from build123d import *

# Parameters (mm, degrees)
F0_R      = 8.25
F1_DEPTH  = 7
F2_R      = 3
F3_DEPTH  = 1
F4_R      = 5.75
F5_DEPTH  = 1.25
F6_R      = 3.35
F7_DEPTH  = 5.5
F9_DEPTH  = 5.5
F10_R     = 2
F11_DEPTH = 25
F13_DEPTH = 2.5


with BuildPart() as f1:
    # F0 (on Top) → F1 (new body)
    with BuildSketch(Plane.XY):
        Circle(F0_R)
    extrude(amount=F1_DEPTH)

    # F2 (on face) → F3 (join)
    with BuildSketch(Plane(origin=(0, 0, 0), x_dir=(1, 0, 0), z_dir=(0, 0, -1))):
        Circle(F2_R)
    extrude(amount=F3_DEPTH)

    # F4 (on face) → F5 (join)
    with BuildSketch(Plane.XY.offset(7)):
        Circle(F4_R)
    extrude(amount=F5_DEPTH)

    # F6 (on face) → F7 (join)
    with BuildSketch(Plane.XY.offset(8.25)):
        Circle(F6_R)
    extrude(amount=F7_DEPTH)

    # F8 (on face) → F9 (cut, through all)
    with BuildSketch(Plane.XY.offset(13.75)):
        with BuildLine():
            ThreePointArc((-2.9, 1.677051), (-3.35, 0), (-2.9, -1.677051))
            Line((-2.9, -1.677051), (-2.9, 1.677051))
        make_face()
        with BuildLine():
            Line((2.9, 1.677051), (2.9, -1.677051))
            ThreePointArc((2.9, -1.677051), (3.235545, -0.868188), (3.35, 0))
            ThreePointArc((3.35, 0), (3.235545, 0.868188), (2.9, 1.677051))
        make_face()
    extrude(amount=-F9_DEPTH, mode=Mode.SUBTRACT)

    # F10 (on face) → F11 (join)
    with BuildSketch(Plane.XY.offset(13.75)):
        Circle(F10_R)
    extrude(amount=F11_DEPTH)

    # F12 (on face) → F13 (join)
    with BuildSketch(Plane.XY.offset(7)):
        Polygon((-8.5, -11.45), (8.5, -11.45), (8.5, -6.003058), (6.946942, -4.45), (-6.946942, -4.45), (-8.5, -6.003058), align=None)
    extrude(amount=-F13_DEPTH)


solid = f1.part
Read the model definition and answer for the solid it produces. Units are mm, in the model's axes. A direction names the side the tool comes from. Coordinates: 2 decimals unless noted, no trailing zeros. Loops run counter-clockwise (first coordinate to the right, second up) from the corner with the lowest first, then second, coordinate; pieces in that order, holes last. Notation, with made-up numbers: (88.5, 14.5) -> (131.5, 14.5) arc R19 cw to (131.5, 43.5) -> close; hole circle Ø6 at (-19.75, 49). An arc over 180 degrees is marked (long way). Answer in a Markdown table with one row per item.
Item 1: A cutting plane is placed at C-C on x = 0. Determine the outline of the cut face in (y, z), plus the area to 3 significant figures.
Returned:
| item | result |
|---|---|
| outline | (-11.45, 4.5) -> (-8.25, 4.5) -> (-8.25, 0) -> (-3, 0) -> (-3, -1) -> (3, -1) -> (3, 0) -> (8.25, 0) -> (8.25, 7) -> (5.75, 7) -> (5.75, 8.25) -> (3.35, 8.25) -> (3.35, 13.75) -> (2, 13.75) -> (2, 38.75) -> (-2, 38.75) -> (-2, 13.75) -> (-3.35, 13.75) -> (-3.35, 8.25) -> (-5.75, 8.25) -> (-5.75, 7) -> (-11.45, 7) -> close |
| area | 281 mm^2 |
Item 2: A cutting plane is placed at D-D on z = 29. Determine the outline of the cut face in (x, y).
Returned:
| item | result |
|---|---|
| outline | circle Ø4 at (0, 0) |
Item 3: Straight lines are drawn through the part: line 1 along Z through (x, y) = (1.75, 2.5); line 2 along Z through (x, y) = (-5, -8.5); line 3 along X through (y, z) = (0, 9). For each, find the intervals that lie inside material, in ascending order. Write a range as [from, to].
Returned:
| item | result |
|---|---|
| line 1 | z = [0, 13.75] |
| line 2 | z = [4.5, 7] |
| line 3 | x = [-2.9, 2.9] |
Item 4: A cutting plane is placed at B-B on y = 0. Determine the outline of the cut face in (x, z).
Returned:
| item | result |
|---|---|
| outline | (-8.25, 0) -> (-3, 0) -> (-3, -1) -> (3, -1) -> (3, 0) -> (8.25, 0) -> (8.25, 7) -> (5.75, 7) -> (5.75, 8.25) -> (2.9, 8.25) -> (2.9, 13.75) -> (2, 13.75) -> (2, 38.75) -> (-2, 38.75) -> (-2, 13.75) -> (-2.9, 13.75) -> (-2.9, 8.25) -> (-5.75, 8.25) -> (-5.75, 7) -> (-8.25, 7) -> close |
Item 5: Each of these flat-tipped pins is pushed along its axis until it touches: P1, Ø4, axis at x = 1, z = 29, coming from the -Y side; P2, Ø8, axis at x = 2.5, y = -8, coming from the -Z side; P3, Ø1, axis at y = -1, z = 11.5, coming from the -X side. Where does it stop, or does it pass through?
Returned:
| item | result |
|---|---|
| P1 | stops at y = -2 |
| P2 | stops at z = 0 |
| P3 | stops at x = -2.9 |
Item 6: A cutting plane is placed at A-A on x = 7.75. Determine the outline of the cut face in (y, z), plus the area to 3 significant figures.
Returned:
| item | result |
|---|---|
| outline | (-11.45, 4.5) -> (-5.25, 4.5) -> (-5.25, 7) -> (-11.45, 7) -> close; (-2.83, 0) -> (2.83, 0) -> (2.83, 7) -> (-2.83, 7) -> close |
| area | 55.1 mm^2 |
Item 7: For faces 1 (the flat face through (-1, 2, 13.75)), 2 (the flat face through (0, -4, 0)), 3 (the cylindrical face through (0.05, 3.35, 10.96)), 4 (the flat face through (0, -9, 4.5)), determine the directions among +Z, -Z, +X, -X, +Y, -Y from which every point of the face is accessible in a straight line to the end or side of a thin tool.
Returned:
| item | result |
|---|---|
| face 1 | +Z |
| face 2 | -Z |
| face 3 | +Z, +Y |
| face 4 | -Z, -Y |
